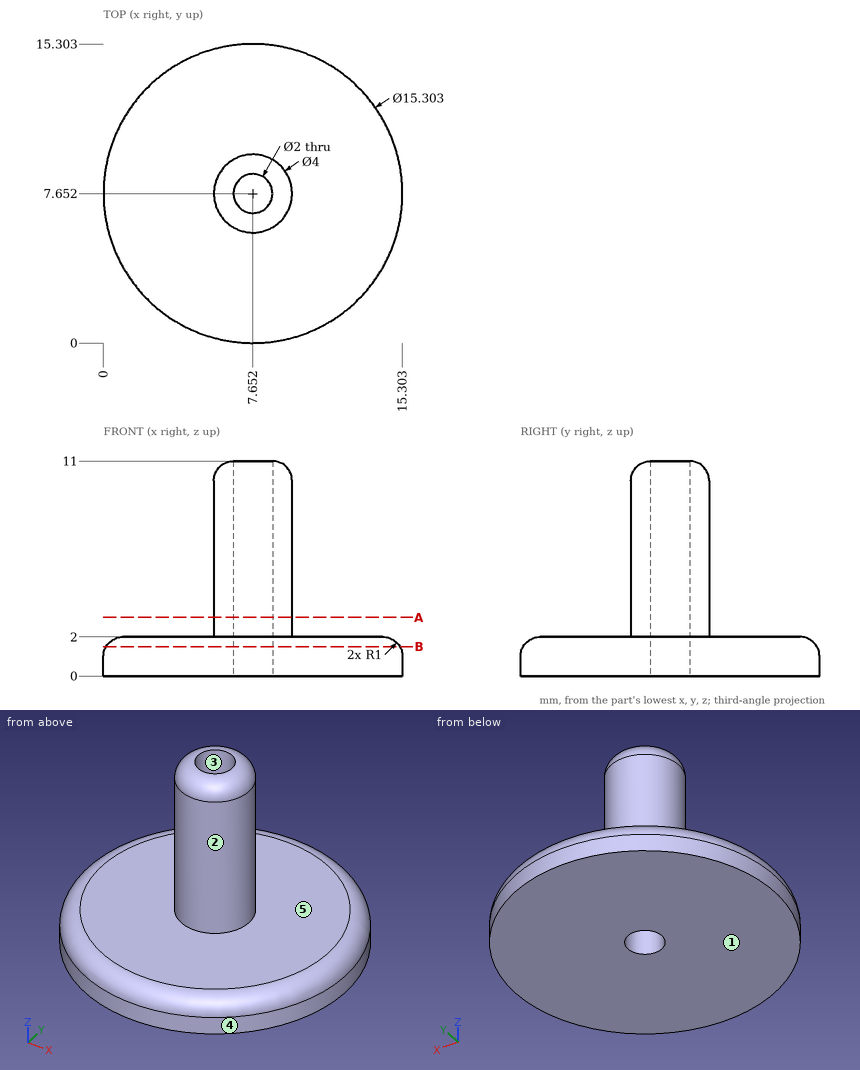
Input: dimensioned drawing with shaded views. Units: mm. Origin: part minimum x, y, z. A direction names the side the tool comes from. Round coordinates to 2 decimals unless told otherwise and drop trailing zeros. Loops run counter-clockwise (first coordinate to the right, second up) from the corner with the lowest first, then second, coordinate; pieces in that order, holes last. Notation, with made-up numbers: (39, 69) -> (83, 69) arc R17 cw to (83, 96) -> close; hole circle Ø11 at (81, 68.25). An arc over 180 degrees is marked (long way). One line per item, written item: value.
(1) Section A-A (z = 3). Return the cut outline in (x, y).
Geometry check:
outline: circle Ø4 at (7.65, 7.65); hole circle Ø2 at (7.65, 7.65)
(2) Set-up query: the marked faces 1 and 2. Return all of +Z, -Z, +X, -X, +Y, -Y with unobstructed straight access to the full face (end or side cutting, diameter ignored); none if empty.
Geometry check:
face 1: -Z, +X, -X, +Y, -Y
face 2: +Z
(3) Mould query, pull axis X, two halves, no side actions, for the marked faces 3, 4 and 5. Classes: pulls with the +X half, pulls with the -X half, needs draft (parallel to the pull), parting line crosses it, or undercut.
Geometry check:
face 3: undercut
face 4: parting line crosses it
face 5: needs draft
(4) Pin query (flat end, axial travel): pin 1 (3 mm diameter, centred on x = 9.5, z = 9, fed in from -Y); pin 2 (2 mm diameter, centred on x = 9.5, z = 1.5, fed in from -Y). Return the tip coordinate at first contact, or that it passes through.
Geometry check:
pin 1: y = 5.68
pin 2: y = 0.06
(5) Material intervals for line 1 (Z direction, x = 3.75, y = 9); line 2 (Y direction, x = 6, z = 8) (1 decimal); line 3 (Y direction, x = 8.75, z = 7) (1 decimal), sorted ascending. Write a range as [from, to].
Geometry check:
line 1: [0, 2]
line 2: [6.5, 8.8]
line 3: [6, 9.3]
(6) Section B-B (z = 1.5). Return the cut outline in (x, y) (1 decimal), plus the area to 3 significant figures.
Geometry check:
outline: circle Ø15 at (7.7, 7.7); hole circle Ø2 at (7.7, 7.7)
area: 174 mm2
